from build123d import *

# Parameters (mm, degrees)
FILLET1_R = 0.5


with BuildPart() as part:
    # Sketch1 → Revolve1 (revolve)
    with BuildSketch(Plane.XY, mode=Mode.PRIVATE) as revolve1_sk:
        with BuildLine():
            Line((7.75, 0), (7.75, 17))
            Line((7.75, 17), (0.712765957, 18.787234043))
            Line((0.712765957, 18.787234043), (0, 19.5))
            Line((0, 19.5), (0, 20))
            Line((0, 20), (0.2, 20))
            ThreePointArc((0.2, 20), (0.268166817, 19.988024693), (0.328170449, 19.95353285))
            Line((0.328170449, 19.95353285), (0.356771445, 19.92965651))
            ThreePointArc((0.356771445, 19.92965651), (0.393979876, 19.905071671), (0.435711125, 19.889343206))
            Line((0.435711125, 19.889343206), (7.996153846, 17.969230769))
            ThreePointArc((7.996153846, 17.969230769), (8.539352217, 17.613940614), (8.75, 17))
            Line((8.75, 17), (8.75, 0))
            Line((8.75, 0), (7.75, 0))
        make_face()
    revolve(revolve1_sk.sketch.rotate(Axis((0, 9.5, 0), (0, -1, 0)), 270), axis=Axis((0, 9.5, 0), (0, -1, 0)))

    # Fillet1
    fillet1_edges = [part.edges().sort_by_distance(p)[0] for p in [
        (0, 0, 8.75),
        (0, 0, 7.75),
    ]]
    fillet(fillet1_edges, radius=FILLET1_R - 0.0001)  # a hair under: the kernel refuses the full size


solid = part.part
Check sheet for the modelled part. Datum: model origin and axes. Units: mm. Round coordinates to 2 decimals unless told otherwise and drop trailing zeros. Write each loop counter-clockwise with the first axis right and the second up, starting at its lowest first coordinate (ties: lowest second). Pieces come first, ordered by that corner, then holes. Notation, with made-up numbers: (-16, 73) - (43, 73) arc R13 cw to (43, 88) - close; hole circle Ø3 at (32, 66). An arc over 180 degrees is marked (long way). Return JSON: item names as keys, results as strings.
Q1. Draft check along Z on faces 1 (the cylindrical face through (7.684, 8.865, 1.009)), 2 (the cylindrical face through (-5.324, 8.634, 6.944)). Enter one of: released by +Z, released by -Z, zero draft, split by the parting line, or undercut.
Returned:
{"face 1": "undercut", "face 2": "split by the parting line"}
Q2. Scan lines: L1, parallel to X at y = 9.5, z = 0; L2, parallel to X at y = 7.75, z = 5; L3, parallel to Z at x = -1.25, y = 14.5. Record each from-to range of solid material in increasing order. Write a range as from..to.
Returned:
{"L1": "x = -8.75..-7.75, 7.75..8.75", "L2": "x = -7.18..-5.92, 5.92..7.18", "L3": "z = -8.66..-7.65, 7.65..8.66"}
Q3. Depth check by flat-ended pin: P1, Ø3, axis at x = -3, y = 10.5, coming from the +Z side; P2, Ø3, axis at x = -3.5, y = 11, coming from the +Z side; P3, Ø1, axis at x = 4, y = 5.5, coming from the +Z side. Enter the tip coordinate at first touch or a pass-through.
Returned:
{"P1": "stops at z = 8.62", "P2": "stops at z = 8.52", "P3": "stops at z = 8.02"}
Q4. Cross-section at A-A (y = 9). Record the boundary of the cut face in (x, z), then the cut area to 3 significant figures.
Returned:
{"outline": "circle Ø17.5 at (0, 0); hole circle Ø15.5 at (0, 0)", "area": "51.8 mm²"}
